from build123d import *

# Parameters (mm, degrees)
SKETCH3_R                = 4.7625
SKETCH3_R_2              = 2.1844
BOSS_EXTRUDE1_DEPTH      = 0.41275
BOSS_EXTRUDE1_DEPTH_BACK = 0.41275
FILLET1_R                = 0.206375


with BuildPart() as part:
    # Sketch3 → Boss-Extrude1 (new body, two sides)
    with BuildSketch(Plane.XY) as boss_extrude1_sk:
        Circle(SKETCH3_R)
        Circle(SKETCH3_R_2, mode=Mode.SUBTRACT)
    extrude(amount=BOSS_EXTRUDE1_DEPTH)
    extrude(boss_extrude1_sk.sketch, amount=-BOSS_EXTRUDE1_DEPTH_BACK)

    # Fillet1
    fillet1_edges = [part.edges().sort_by_distance(p)[0] for p in [
        (-4.7625, 0, 0.41275),
        (-2.1844, 0, 0.41275),
    ]]
    fillet(fillet1_edges, radius=FILLET1_R)


solid = part.part
Could you check a few things on this model? Use its own coordinates, in mm. Coordinates: 2 decimals unless noted, no trailing zeros. Write each loop counter-clockwise with the first axis right and the second up, starting at its lowest first coordinate (ties: lowest second). Pieces come first, ordered by that corner, then holes. Notation, with made-up numbers: (43, 84) - (84, 84) arc R19 cw to (84, 118) - close; hole circle Ø5 at (-19.75, 1.25). An arc over 180 degrees is marked (long way). Put each result on its own line as item: value. Start each with the question number.
Q1. I want a section at A-A on x = 0. Write out the boundary of the cut face in (y, z), plus the area to 3 significant figures.
Q2. Please list where these lines run through material, in increasing order: L1, parallel to Y at x = 0, z = -0.2; L2, parallel to X at y = 0.25, z = -0.2; L3, parallel to X at y = 1, z = -0.2.
Checks:
1. outline: (-4.76, -0.41) - (-2.18, -0.41) - (-2.18, 0.21) arc R0.21 ccw to (-2.39, 0.41) - (-4.56, 0.41) arc R0.21 ccw to (-4.76, 0.21) - close; (2.18, -0.41) - (4.76, -0.41) - (4.76, 0.21) arc R0.21 ccw to (4.56, 0.41) - (2.39, 0.41) arc R0.21 ccw to (2.18, 0.21) - close
1. area: 4.22 mm²
2. L1: -4.76 to -2.18, 2.18 to 4.76
2. L2: -4.76 to -2.17, 2.17 to 4.76
2. L3: -4.66 to -1.94, 1.94 to 4.66
